```python
from build123d import *

# Parameters (mm, degrees)
SKETCH1_R                 = 12.4
BOSS_EXTRUDE2_DEPTH       = 21
SKETCH3_R                 = 12.115
BOSS_EXTRUDE3_DEPTH       = 30.8
SKETCH4_R                 = 12.05
BOSS_EXTRUDE4_DEPTH       = 16.2
SKETCH5_R                 = 3.5
BOSS_EXTRUDE5_DEPTH       = 2.5
BOSS_EXTRUDE6_DEPTH       = 11.25
M3X0_5_TAPPED_HOLE1_D     = 2.5
M3X0_5_TAPPED_HOLE1_DEPTH = 4
M3X0_5_TAPPED_HOLE1_TIP   = 0.751075774
SKETCH9_W                 = 5
SKETCH9_H                 = 13
CUT_EXTRUDE2_DEPTH        = 13.4


with BuildPart() as part:
    # Sketch1 → Boss-Extrude2 (new body)
    with BuildSketch(Plane(origin=(0, 0, 0), x_dir=(0, 0, -1), z_dir=(1, 0, 0))):
        Circle(SKETCH1_R)
    extrude(amount=-BOSS_EXTRUDE2_DEPTH)

    # Sketch3 → Boss-Extrude3 (add)
    with BuildSketch(Plane.ZY.offset(21)):
        Circle(SKETCH3_R)
    extrude(amount=BOSS_EXTRUDE3_DEPTH)

    # Sketch4 → Boss-Extrude4 (add)
    with BuildSketch(Plane.ZY.offset(51.8)):
        Circle(SKETCH4_R)
    extrude(amount=BOSS_EXTRUDE4_DEPTH)

    # Sketch5 → Boss-Extrude5 (add)
    with BuildSketch(Plane(origin=(0, 0, 0), x_dir=(0, 0, -1), z_dir=(1, 0, 0))):
        Circle(SKETCH5_R)
    extrude(amount=BOSS_EXTRUDE5_DEPTH)

    # Sketch6 → Boss-Extrude6 (add)
    with BuildSketch(Plane(origin=(2.5, 0, 0), x_dir=(0, 0, -1), z_dir=(1, 0, 0))):
        with BuildLine():
            Line((-1.322875656, 1.5), (1.322875656, 1.5))
            ThreePointArc((1.322875656, 1.5), (0, -2), (-1.322875656, 1.5))
        make_face()
    extrude(amount=BOSS_EXTRUDE6_DEPTH)

    # M3x0.5 Tapped Hole1
    with Locations(Plane(origin=(0, 0, 0), x_dir=(0, 0, -1), z_dir=(1, 0, 0))):
        with Locations((-8.5, 0), (8.5, 0)):
            Hole(M3X0_5_TAPPED_HOLE1_D / 2, depth=M3X0_5_TAPPED_HOLE1_DEPTH)
            with Locations((0, 0, -(M3X0_5_TAPPED_HOLE1_DEPTH + M3X0_5_TAPPED_HOLE1_TIP / 2))):  # 118° drill point
                Cone(0, M3X0_5_TAPPED_HOLE1_D / 2, M3X0_5_TAPPED_HOLE1_TIP, mode=Mode.SUBTRACT)

    # Sketch9 → Cut-Extrude2 (cut, through all)
    with BuildSketch(Plane.XY):
        with Locations((-56.3, 0)):
            Rectangle(SKETCH9_W, SKETCH9_H)
    extrude(amount=CUT_EXTRUDE2_DEPTH, mode=Mode.SUBTRACT)


solid = part.part
```
Input: part model. Units: mm. Frame: model coordinates. A direction names the side the tool comes from. Give positions to 0.01 mm unless a question says otherwise; leave off trailing zeros. Order: outer loops, then holes, each group sorted by start corner. A loop starts at its lowest first (then second) coordinate and runs counter-clockwise, first axis right, second up. Notation, with made-up numbers: (34.25, 6) - (85.25, 6) arc R8 ccw to (85.25, 12) - close; hole circle Ø5 at (-1, -17.75). An arc over 180 degrees is marked (long way). One line per item, written item: value.
1. Cut plane B-B, the plane y = 5.5. Output: boundary loops of the cut face in (x, z), and give its area (3 significant figures).
Determined:
outline: (-68, -10.72) - (-51.8, -10.72) - (-51.8, -10.79) - (-21, -10.79) - (-21, -11.11) - (0, -11.11) - (0, 11.11) - (-21, 11.11) - (-21, 10.79) - (-51.8, 10.79) - (-51.8, 10.72) - (-53.8, 10.72) - (-53.8, 0) - (-58.8, 0) - (-58.8, 10.72) - (-68, 10.72) - close
area: 1,430 mm2
2. Reachability of faces 1 (the face through (8, -2, 0)), 2 (the face through (-59.79, 0.53, -12.04)), 3 (the face through (-56, 6.5, 5)) from +Z, -Z, +X, -X, +Y, -Y: full face, straight path, thin tool, end or side. Return the list, or none.
Determined:
face 1: +X
face 2: -X
face 3: +Z
3. Draft query along Y for faces 4 (the face through (-56, -6.5, 5)), 5 (the face through (-36.184, -11.827, -2.626)), 6 (the face through (13.75, 0, 0)). Return one class per face: released by +Y, released by -Y, zero draft, split by the parting line, or undercut.
Determined:
face 4: undercut
face 5: split by the parting line
face 6: zero draft
4. Line query: probe 1 along X at (y, z) = (-3.5, 6.25); probe 2 along X at (y, z) = (2.5, -6.5); probe 3 along Y at (x, z) = (-2.5, -8.5). Output: solid intervals per line, ascending.
Determined:
probe 1: -68 to -58.8, -53.8 to 0
probe 2: -68 to 0
probe 3: -9.03 to -1.25, 1.25 to 9.03
5. Cut plane C-C, the plane z = 4.75. Output: boundary loops of the cut face in (x, y), and give its area (3 significant figures).
Determined:
outline: (-68, -11.07) - (-51.8, -11.07) - (-51.8, -11.14) - (-21, -11.14) - (-21, -11.45) - (0, -11.45) - (0, 11.45) - (-21, 11.45) - (-21, 11.14) - (-51.8, 11.14) - (-51.8, 11.07) - (-68, 11.07) - close; hole (-58.8, -6.5) - (-53.8, -6.5) - (-53.8, 6.5) - (-58.8, 6.5) - close
area: 1,460 mm2
6. Cut plane A-A, the plane z = -4.5. Output: boundary loops of the cut face in (x, y).
Determined:
outline: (-68, -11.18) - (-51.8, -11.18) - (-51.8, -11.25) - (-21, -11.25) - (-21, -11.55) - (0, -11.55) - (0, 11.55) - (-21, 11.55) - (-21, 11.25) - (-51.8, 11.25) - (-51.8, 11.18) - (-68, 11.18) - close
7. Pin query (flat end, axial travel): pin 1 Ø1 at (x, y) = (-27, -9) entering from -Z; pin 2 Ø1 at (x, z) = (-6.5, 9) entering from -Y; pin 3 Ø5.5 at (x, y) = (-55, 0.5) entering from +Z. Return the tip coordinate at first contact, or that it passes through.
Determined:
pin 1: z = -8.63
pin 2: y = -9.03
pin 3: z = 12.05
8. Cut plane D-D, the plane x = -48. Output: boundary loops of the cut face in (y, z) (3 decimals).
Determined:
outline: circle Ø24.23 at (0, 0)
